Autodesk Inventor part; units mm, degrees
ref_plane "YZ Plane" through (0, 0, 0) normal (1, 0, 0) x (0, 1, 0)
ref_plane "XY Plane" through (0, 0, 0) normal (0, 0, 1) x (1, 0, 0)
sketch "Sketch1" plane through (0, 0, 0) normal (0, 0, 1) x (1, 0, 0)
  line L0 (-22, 38.0007) -> (21.9822, 38.0007)
  line L1 (21.9822, 38.0007) -> (21.9822, -66)
  line L2 (-22, -66) -> (-22, 38.0007)
  arc A0 (-22, -65.3741) -> (21.9822, -65.3741) centre (-0.0089, -66) ccw
  point P0 (0, 0)
  dimension "d22" = 44
extrude "Extrusion1" add sketch "Sketch1" along normal blind 4
sketch "Sketch2" plane through (0, 0, 0) normal (0, 0, 1) x (1, 0, 0)
  circle A0 centre (-15.5, 31.5) radius 2
  circle A1 centre (15.5, 31.5) radius 2
  circle A2 centre (-15.5, -0.5) radius 2
  circle A3 centre (15.5, -0.5) radius 2
  point P0 (0, 0)
extrude "Extrusion2" cut sketch "Sketch2" along normal blind 4
sketch "Sketch3" plane through (0, 0, 0) normal (0, 0, 1) x (1, 0, 0)
  circle A0 centre (0, -78) radius 2.5
  point P0 (0, 0)
  dimension "d24" = 5
extrude "Extrusion3" cut sketch "Sketch3" along normal blind 4
ref_plane "Work Plane1" through (0, -60, 0) normal (0, 1, 0) x (-1, 0, 0)
sketch "Sketch4" plane through (0, -60, 0) normal (0, 1, 0) x (-1, 0, 0)
  circle A0 centre (0, 4) radius 2
  point P0 (0, 0)
  dimension "d14" = 4
extrude "Extrusion4" cut sketch "Sketch4" along normal blind 51.75 and the other way blind 11.25
sketch "Sketch5" plane through (0, 0, 4) normal (0, 0, 1) x (1, 0, 0)
  circle A0 centre (0, 16.6667) radius 12.5
  point P0 (0, 0)
  dimension "d19" = 25
extrude "Extrusion5" cut sketch "Sketch5" against normal blind 4
properties part number "DispenserBrace"
Can you work these out from the model? Positions are in its coordinate system, mm. A direction names the side the tool comes from. Give positions to 0.01 mm unless a question says otherwise; leave off trailing zeros. Loops run counter-clockwise (first coordinate to the right, second up) from the corner with the lowest first, then second, coordinate; pieces in that order, holes last. Notation, with made-up numbers: M -7,-6.75 L 41,-6.75 A30 ccw 41,21.25 Z; hole C 59.5,53 d1. An arc over 180 degrees is marked long. Answer in a Markdown table with one row per item.
1. If I drill on line 1 along Y through (x, z) = (-15.5, 1.55); line 2 along Y through (x, z) = (-2, 1.95); line 3 along X through (y, z) = (8, 2.8), over which ranges is the centre line in solid material (lowest first)?
Taken from the geometry:
| item | result |
|---|---|
| line 1 | y = -81.62 to -2.5, 1.5 to 29.5, 33.5 to 38 |
| line 2 | y = -87.91 to -79.5, -76.5 to 4.33, 29.01 to 38 |
| line 3 | x = -22 to -9.01, 9.01 to 21.98 |
2. For pin 1 Ø2 at (y, z) = (9, 2.5) entering from +X; pin 2 Ø3.5 at (x, y) = (15.5, -0.5) entering from -Z; pin 3 Ø0.6 at (x, z) = (0, 2.5) entering from -Y; pin 4 Ø1.2 at (y, z) = (-38.5, 2.5) entering from -X, each with a flat end and sliding along its axis, tell me the tip position at first contact or that it passes through.
Taken from the geometry:
| item | result |
|---|---|
| pin 1 | stops at x = 21.98 |
| pin 2 | passes through |
| pin 3 | stops at y = -88 |
| pin 4 | stops at x = -22 |
3. Suppose I cut it at C-C on x = 11. Write out the boundary of the cut face in (y, z), plus the area to 3 significant figures.
Taken from the geometry:
| item | result |
|---|---|
| outline | M -85.05,0 L 10.73,0 L 10.73,4 L -85.05,4 Z; M 22.6,0 L 38,0 L 38,4 L 22.6,4 Z |
| area | 445 mm² |
4. Suppose I cut it at D-D on y = 15. Write out the boundary of the cut face in (x, z).
Taken from the geometry:
| item | result |
|---|---|
| outline | M -22,0 L -12.39,0 L -12.39,4 L -22,4 Z; M 12.39,0 L 21.98,0 L 21.98,4 L 12.39,4 Z |
5. Thinking about a two-plate mould opening in Y: for faces 3 (the flat face through (21.982, -13, 2)), 4 (the cylindrical face through (-15.934, 33.452, 1.972)), 5 (the flat face through (0, 38.001, 2)), which applies, released by +Y, released by -Y, zero draft, split by the parting line, or undercut?
Taken from the geometry:
| item | result |
|---|---|
| face 3 | zero draft |
| face 4 | undercut |
| face 5 | released by +Y |
6. Suppose I cut it at A-A on y = -0.5. Write out the boundary of the cut face in (x, z), plus the area to 3 significant figures.
Taken from the geometry:
| item | result |
|---|---|
| outline | M -22,0 L -17.5,0 L -17.5,4 L -22,4 Z; M -13.5,0 L 13.5,0 L 13.5,4 L -13.5,4 Z; M 17.5,0 L 21.98,0 L 21.98,4 L 17.5,4 Z |
| area | 144 mm² |
7. Which directions (+Z, -Z, +X, -X, +Y, -Y) give clear straight access to the entire face, cutting with the end or side of a thin tool? Please do faces 1 (the cylindrical face through (0, -39, 2)), 2 (the cylindrical face through (15.066, 33.452, 1.972)).
Taken from the geometry:
| item | result |
|---|---|
| face 1 | +Z |
| face 2 | +Z, -Z |
8. Suppose I cut it at B-B on x = -15.5. Write out the boundary of the cut face in (y, z).
Taken from the geometry:
| item | result |
|---|---|
| outline | M -81.62,0 L -2.5,0 L -2.5,4 L -81.62,4 Z; M 1.5,0 L 29.5,0 L 29.5,4 L 1.5,4 Z; M 33.5,0 L 38,0 L 38,4 L 33.5,4 Z |
